Print and shaded views of the part. All mm, measured from the part's lowest x, y and z. A direction names the side the tool comes from. Coordinates: 2 decimals unless noted, no trailing zeros. Write each loop counter-clockwise with the first axis right and the second up, starting at its lowest first coordinate (ties: lowest second). Pieces come first, ordered by that corner, then holes. Notation, with made-up numbers: (47.25, -23) -> (64.25, -23) arc R30 cw to (64.25, -1) -> close; hole circle Ø3 at (44, -28.75). An arc over 180 degrees is marked (long way). Write item = value, one per line.
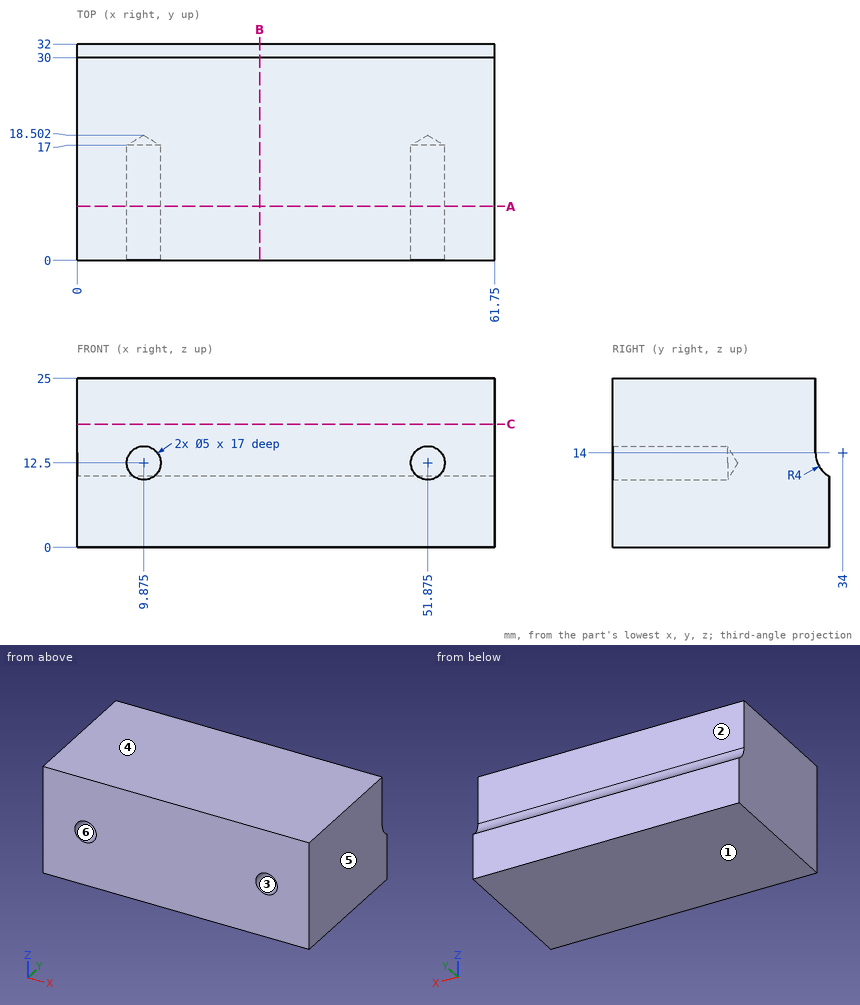
Q1. Mould opens along Z. For the marked faces 4, 5 and 6 say: released by +Z, released by -Z, zero draft, split by the parting line, or undercut.
Model answer:
face_4 = released by +Z
face_5 = zero draft
face_6 = undercut
Q2. Saw through at A-A on y = 8. Give the cut face in (x, z) (3 decimals), and give its area (3 significant figures).
Model answer:
outline = (0, 0) -> (61.75, 0) -> (61.75, 25) -> (0, 25) -> close; hole circle Ø5 at (9.875, 12.5); hole circle Ø5 at (51.875, 12.5)
area = 1,500 mm²
Q3. Which spindle directions (+Z, -Z, +X, -X, +Y, -Y) get a long thin tool onto all of the face, cutting with end or side? Do the marked faces 1, 2 and 3. Say none if no direction does.
Model answer:
face_1 = -Z, +X, -X, +Y, -Y
face_2 = +Z, +X, -X, +Y
face_3 = -Y
Q4. Probe line 1 (X direction, y = 7, z = 12.5) (3 decimals); line 2 (Y direction, x = 14, z = 14); line 3 (Z direction, x = 52, y = 18) (1 decimal). List the from-to ranges inside material, lowest first. Write a range as from..to.
Model answer:
line_1 = 0..7.375, 12.375..49.375, 54.375..61.75
line_2 = 0..30
line_3 = 0..11.7, 13.3..25
Q5. Saw through at C-C on z = 18.25. Give the cut face in (x, y), and give its area (3 significant figures).
Model answer:
outline = (0, 0) -> (61.75, 0) -> (61.75, 30) -> (0, 30) -> close
area = 1,850 mm²
Q6. Pin check, flat tips, straight feed: pin 1 (8 mm diameter, centred on y = 28.5, z = 9.5, fed in from -X); pin 2 (12 mm diameter, centred on x = 19.5, z = 21.5, fed in from +Y). Stop position of each tip, or through.
Model answer:
pin_1 = 0
pin_2 = 30
Q7. Saw through at B-B on x = 27. Give the cut face in (y, z).
Model answer:
outline = (0, 0) -> (32, 0) -> (32, 10.54) arc R4 cw to (30, 14) -> (30, 25) -> (0, 25) -> close
